from build123d import *

# Parameters (mm, degrees)
ESQUISSE1_W        = 120
ESQUISSE1_H        = 15
ESQUISSE1_R        = 2
BOSS_EXTRU_1_DEPTH = 5
CONG_1_R           = 3


with BuildPart() as part:
    # Esquisse1 → Boss.-Extru.1 (new body)
    with BuildSketch(Plane.XY):
        Rectangle(ESQUISSE1_W, ESQUISSE1_H)
        with Locations((-55, 0)):
            Circle(ESQUISSE1_R, mode=Mode.SUBTRACT)
        with Locations(Location((55, 0, 0), (0, 0, 180))):
            Circle(ESQUISSE1_R, mode=Mode.SUBTRACT)
    extrude(amount=BOSS_EXTRU_1_DEPTH)

    # Congé1
    cong_1_edges = [part.edges().sort_by_distance(p)[0] for p in [
        (60, -7.5, 2.5),
        (-60, -7.5, 2.5),
        (-60, 7.5, 2.5),
        (60, 7.5, 2.5),
    ]]
    fillet(cong_1_edges, radius=CONG_1_R)


solid = part.part
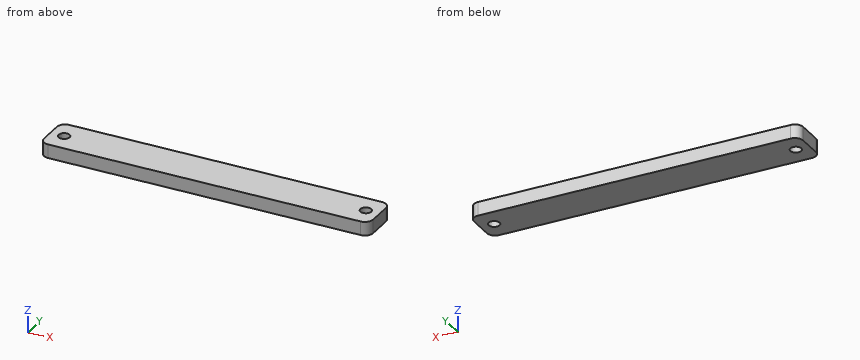
Work out the finished part from the listing and answer in its coordinate system (mm). Give positions to 0.01 mm unless a question says otherwise; leave off trailing zeros. Loops run counter-clockwise (first coordinate to the right, second up) from the corner with the lowest first, then second, coordinate; pieces in that order, holes last. Notation, with made-up numbers: (30, 59.25) - (53, 59.25) arc R21 ccw to (53, 67.25) - close; hole circle Ø7 at (52.5, -5). An arc over 180 degrees is marked (long way). Answer in a Markdown table with one row per item.
(1) A flat-ended cylindrical pin translates along its axis: pin 1 Ø3.5 at (x, y) = (-55, 0) entering from +Z. Find the tip coordinate at first contact, or state that the pin passes through.
Results list:
| item | result |
|---|---|
| pin 1 | passes through |
(2) Section A-A (z = 2.85) is taken. Give the vertices of the cut face in (x, y).
Results list:
| item | result |
|---|---|
| outline | (-60, -4.5) arc R3 ccw to (-57, -7.5) - (57, -7.5) arc R3 ccw to (60, -4.5) - (60, 4.5) arc R3 ccw to (57, 7.5) - (-57, 7.5) arc R3 ccw to (-60, 4.5) - close; hole circle Ø4 at (-55, 0); hole circle Ø4 at (55, 0) |
(3) Consider L1, parallel to Y at x = -55, z = 1.7; L2, parallel to X at y = -0.5, z = 1.65; L3, parallel to X at y = -1.5, z = 0.7. Determine where each line is inside the solid, lowest interval first. Write a range as [from, to].
Results list:
| item | result |
|---|---|
| L1 | y = [-7.5, -2], [2, 7.5] |
| L2 | x = [-60, -56.94], [-53.06, 53.06], [56.94, 60] |
| L3 | x = [-60, -56.32], [-53.68, 53.68], [56.32, 60] |
(4) Section C-C (x = 55) is taken. Give the vertices of the cut face in (y, z).
Results list:
| item | result |
|---|---|
| outline | (-7.5, 0) - (-2, 0) - (-2, 5) - (-7.5, 5) - close; (2, 0) - (7.5, 0) - (7.5, 5) - (2, 5) - close |
(5) Section B-B (y = 0) is taken. Give the vertices of the cut face in (x, z), and give its area (3 significant figures).
Results list:
| item | result |
|---|---|
| outline | (-60, 0) - (-57, 0) - (-57, 5) - (-60, 5) - close; (-53, 0) - (53, 0) - (53, 5) - (-53, 5) - close; (57, 0) - (60, 0) - (60, 5) - (57, 5) - close |
| area | 560 mm² |
